```python
from build123d import *

# Parameters (mm, degrees)
SKETCH5_R           = 38.5
BOSS_EXTRUDE2_DEPTH = 6.36
SKETCH7_R           = 3.5
CUT_EXTRUDE3_DEPTH  = 1086.328407818
SKETCH8_R           = 11
CUT_EXTRUDE4_DEPTH  = 1086.328407818


with BuildPart() as part:
    # Sketch5 → Boss-Extrude2 (new body)
    with BuildSketch(Plane(origin=(0, 0, 0), x_dir=(1, 0, 0), z_dir=(0, 1, 0))):
        with Locations(Location((933.152542373, 445.016949153, 0), (0, 0, 90))):
            Circle(SKETCH5_R)
    extrude(amount=BOSS_EXTRUDE2_DEPTH)

    # Sketch7 → Cut-Extrude3 (cut, through all)
    with BuildSketch(Plane(origin=(0, 6.36, 0), x_dir=(1, 0, 0), z_dir=(0, 1, 0))):
        with Locations(Location((933.152542373, 475.016949153, 0), (0, 0, 270))):
            Circle(SKETCH7_R)
        with Locations((-55.199525992, -1045.642281877)):
            Circle(SKETCH7_R)
        with Locations((-877.953016381, 570.625332725)):
            Circle(SKETCH7_R)
        with Locations(Location((959.133304486, 430.016949153, 0), (0, 0, 270))):
            Circle(SKETCH7_R)
        with Locations(Location((907.171780259, 430.016949153, 0), (0, 0, 270))):
            Circle(SKETCH7_R)
    extrude(amount=-CUT_EXTRUDE3_DEPTH, mode=Mode.SUBTRACT)

    # Sketch8 → Cut-Extrude4 (cut, through all)
    with BuildSketch(Plane(origin=(0, 6.36, 0), x_dir=(1, 0, 0), z_dir=(0, 1, 0))):
        with Locations(Location((933.152542373, 445.016949153, 0), (0, 0, 270))):
            Circle(SKETCH8_R)
    extrude(amount=-CUT_EXTRUDE4_DEPTH, mode=Mode.SUBTRACT)


solid = part.part
```
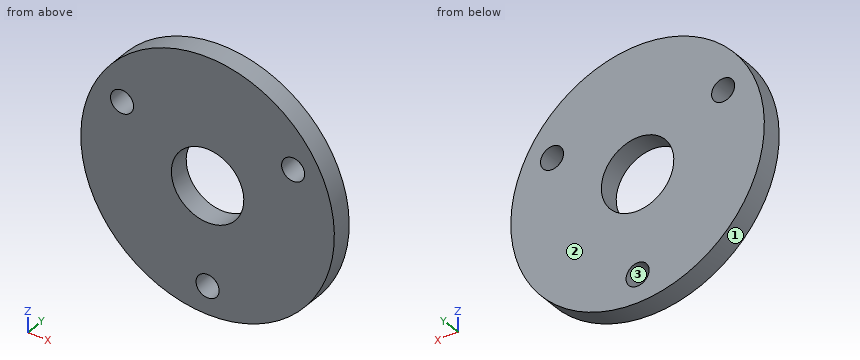
Design review of the part built by this model. Coordinates are the model's own, in mm. Face numbers are marked on the shaded views. Give positions to 0.01 mm unless a question says otherwise; leave off trailing zeros. Order: outer loops, then holes, each group sorted by start corner. A loop starts at its lowest first (then second) coordinate and runs counter-clockwise, first axis right, second up. Notation, with made-up numbers: M 85.5,52.25 L 89.5,52.25 A15 cw 89.5,56.25 Z; hole C -19,-8.5 d6. An arc over 180 degrees is marked long. One line per question, with ' | ' between items. Start each with the question number.
Q1. For L1, parallel to Z at x = 933.5, y = 5; L2, parallel to X at y = 3.5, z = -430.5; L3, parallel to Z at x = 909, y = 4.5, list the stretches that pass through material, from the lowest coordinate up. Write a range as [from, to].
Q2. The part is to be moulded in two halves that separate along Z. For the marked faces 1, 2 and 3, say which applies: +Z half, -Z half, draft (parallel to the pull), parting line (faces both ways), or undercut.
Q3. We need section B-B (y = 1.25). Write out the cut boundary in (x, z).
Q4. We need section D-D (x = 902.5). Write out the cut boundary in (y, z), plus the area to 3 significant figures.
Q5. For pin 1 Ø2 at (y, z) = (2, -434) entering from -X; pin 2 Ø1.5 at (y, z) = (1, -434) entering from -X; pin 3 Ø2 at (x, y) = (961.5, 3.5) entering from +Z, all flat-tipped, find the tip position at first contact; note any pin that passes through.
Q6. We need section A-A (z = -475). Write out the cut boundary in (x, y), plus the area to 3 significant figures.
Q7. We need section C-C (z = -436). Write out the cut boundary in (x, y), plus the area to 3 significant figures.
Returned:
1) L1: [-483.52, -478.5], [-471.53, -456.01], [-434.02, -406.52] | L2: [897.49, 903.71], [910.64, 955.67], [962.6, 968.81] | L3: [-475, -433], [-427.03, -415.04]
2) face 1: parting line | face 2: draft | face 3: undercut
3) outline: C 933.15,-445.02 d77; hole C 907.17,-430.02 d7; hole C 933.15,-445.02 d22; hole C 933.15,-475.02 d7; hole C 959.13,-430.02 d7
4) outline: M 0,-468.31 L 6.36,-468.31 L 6.36,-421.72 L 0,-421.72 Z | area: 296 mm2
5) pin 1: x = 895.98 | pin 2: x = 896.05 | pin 3: z = -417.92
6) outline: M 909,0 L 929.65,0 L 929.65,6.36 L 909,6.36 Z; M 936.65,0 L 957.3,0 L 957.3,6.36 L 936.65,6.36 Z | area: 263 mm2
7) outline: M 895.72,0 L 926.85,0 L 926.85,6.36 L 895.72,6.36 Z; M 939.45,0 L 970.58,0 L 970.58,6.36 L 939.45,6.36 Z | area: 396 mm2
